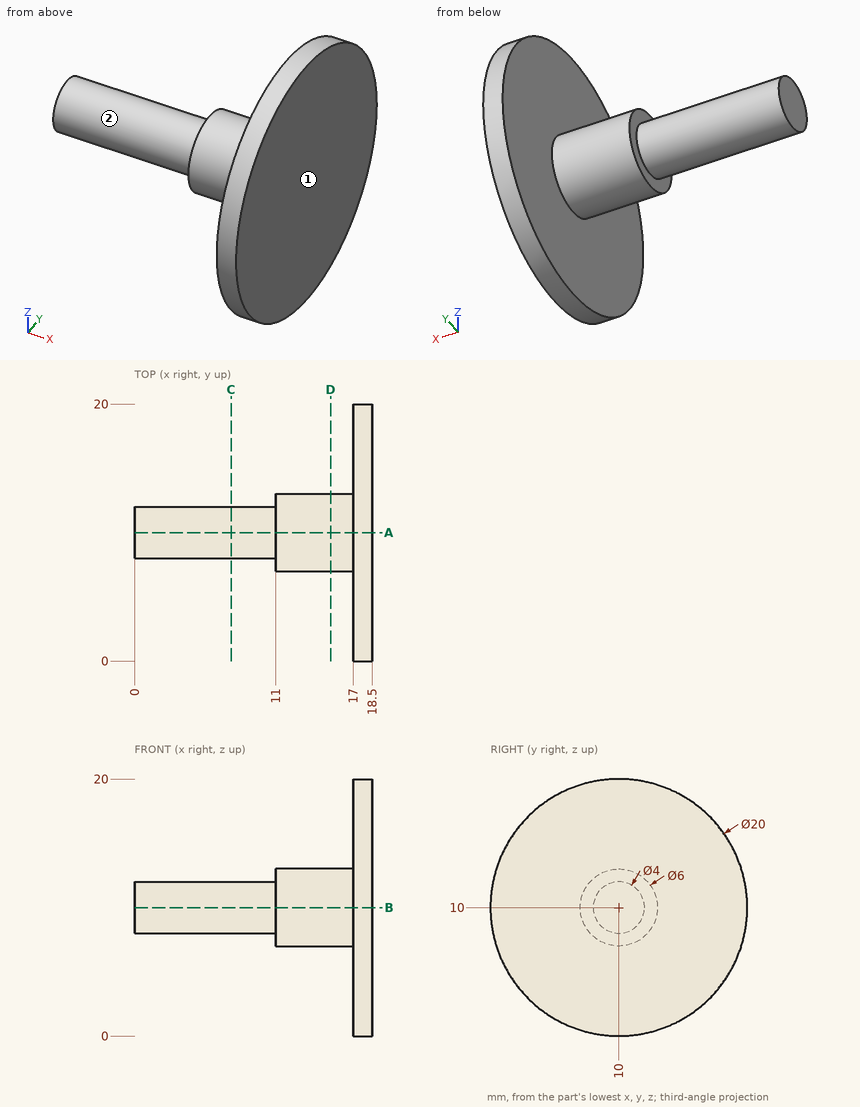
Can you work these out from the drawing? Everything is in mm from the part's minimum corner. A direction names the side the tool comes from. Give positions to 0.01 mm unless a question says otherwise; leave off trailing zeros. Loops run counter-clockwise (first coordinate to the right, second up) from the corner with the lowest first, then second, coordinate; pieces in that order, holes last. Notation, with made-up numbers: (82.25, 32) -> (135.25, 32) arc R25 ccw to (135.25, 67) -> close; hole circle Ø6 at (-21, 58.5). An arc over 180 degrees is marked (long way). Return JSON: item names as keys, results as strings.
Item 1: I need wall thicknesses on L1, parallel to X at y = 18.5, z = 5.5; L2, parallel to Z at x = 16.5, y = 8.25; L3, parallel to Z at x = 13.5, y = 7.25. Which ranges of each line are inside material? Lowest first, please. Write a range as from..to.
Geometry results:
{"L1": "x = 17..18.5", "L2": "z = 7.56..12.44", "L3": "z = 8.8..11.2"}
Item 2: If we section it at D-D on x = 15.25: List the corners of the cut face in (y, z) for me, plus the area to 3 significant figures.
Geometry results:
{"outline": "circle Ø6 at (10, 10)", "area": "28.3 mm²"}
Item 3: If we section it at A-A on y = 10: List the corners of the cut face in (x, z) for me, plus the area to 3 significant figures.
Geometry results:
{"outline": "(0, 8) -> (11, 8) -> (11, 7) -> (17, 7) -> (17, 0) -> (18.5, 0) -> (18.5, 20) -> (17, 20) -> (17, 13) -> (11, 13) -> (11, 12) -> (0, 12) -> close", "area": "110 mm²"}
Item 4: If we section it at C-C on x = 7.5: List the corners of the cut face in (y, z) for me.
Geometry results:
{"outline": "circle Ø4 at (10, 10)"}
Item 5: Which directions (+Z, -Z, +X, -X, +Y, -Y) give clear straight access to the entire face, cutting with the end or side of a thin tool? Please do the marked faces 1 and 2.
Geometry results:
{"face 1": "+Z, -Z, +X, +Y, -Y", "face 2": "-X"}
Item 6: I'm going to push flat-ended pins straight in: pin 1 (1.5 mm diameter, centred on y = 10.5, z = 16.5, fed in from -X); pin 2 (3 mm diameter, centred on x = 5.5, y = 12.5, fed in from -Z). Where does each tip first touch, or does it pass through?
Geometry results:
{"pin 1": "stops at x = 17", "pin 2": "stops at z = 8.27"}
